Source: CAD feature listing. Evaluate the final solid. Frame: model axes, mm. A direction names the side the tool comes from. Give positions to 0.01 mm unless a question says otherwise; leave off trailing zeros. Loops run counter-clockwise (first coordinate to the right, second up) from the corner with the lowest first, then second, coordinate; pieces in that order, holes last. Notation, with made-up numbers: M 40.25,60 L 47.25,60 A23 ccw 47.25,76 Z; hole C 70,-17 d6. An arc over 180 degrees is marked long. Write item = value, one per line.
Autodesk Inventor part; units mm, degrees
ref_plane "YZ Plane" through (0, 0, 0) normal (1, 0, 0) x (0, 1, 0)
ref_plane "XZ Plane" through (0, 0, 0) normal (0, 1, 0) x (-1, 0, 0)
ref_plane "XY Plane" through (0, 0, 0) normal (0, 0, 1) x (1, 0, 0)
sketch "Sketch1" plane through (0, 0, 0) normal (0, 0, 1) x (1, 0, 0)
  line L0 (-25, 25) -> (25, 25)
  line L1 (25, 25) -> (25, -25)
  line L2 (25, -25) -> (-25, -25)
  line L3 (-25, -25) -> (-25, 25)
  line L4 (-25, 25) -> (25, -25) construction
  line L5 (25, 25) -> (-25, -25) construction
  circle A0 centre (0, 0) radius 2.5
  circle A1 centre (-20.8, -14.5) radius 2.65
  circle A2 centre (-14.5, -20.8) radius 2.65
  circle A3 centre (-20.8, 14.5) radius 2.65
  circle A4 centre (20.8, -14.5) radius 2.65
  circle A5 centre (20.8, 14.5) radius 2.65
  circle A6 centre (-14.5, 20.8) radius 2.65
  circle A7 centre (14.5, -20.8) radius 2.65
  circle A8 centre (14.5, 20.8) radius 2.65
  dimension "d0" = 50
  dimension "d1" = 50
  dimension "d2" = 5
  dimension "d5" = 5.3
  dimension "d6" = 4.2
  dimension "d8" = 10.5
  dimension "d11" = 29
  dimension "d14" = 41.6
extrude "Extrusion1" add sketch "Sketch1" along normal blind 5
fillet "Fillet1" radius 2 4 edges at (-25, 25, 2.5) (25, 25, 2.5) (-25, -25, 2.5) (25, -25, 2.5)
sketch "Sketch2" plane through (0, 0, 5) normal (0, 0, 1) x (1, 0, 0)
  arc A0 (23, -25) -> (25, -23) centre (23, -23) ccw
  line L0 (25, -23) -> (25, 23)
  arc A1 (25, 23) -> (23, 25) centre (23, 23) ccw
  line L1 (23, 25) -> (-23, 25)
  arc A2 (-23, 25) -> (-25, 23) centre (-23, 23) ccw
  line L2 (-25, 23) -> (-25, -23)
  arc A3 (-25, -23) -> (-23, -25) centre (-23, -23) ccw
  line L3 (-23, -25) -> (23, -25)
  circle A4 centre (14.5, 20.8) radius 2.65
  circle A5 centre (-14.5, 20.8) radius 2.65
  circle A6 centre (14.5, -20.8) radius 2.65
  circle A7 centre (20.8, 14.5) radius 2.65
  circle A8 centre (20.8, -14.5) radius 2.65
  circle A9 centre (-20.8, 14.5) radius 2.65
  circle A10 centre (-14.5, -20.8) radius 2.65
  circle A11 centre (-20.8, -14.5) radius 2.65
  circle A12 centre (0, 0) radius 2.5
  line L4 (21, -21) -> (-21, -21)
  line L5 (-21, -21) -> (-21, 21)
  line L6 (-21, 21) -> (21, 21)
  line L7 (21, 21) -> (21, -21)
  line L8 (21, -21) -> (-21, 21) construction
  line L9 (-21, -21) -> (21, 21) construction
  circle A13 centre (-28.6, 21.06) radius 1.55
  dimension "d18" = 42
  dimension "d19" = 42
hole "Hole1" at (-21, 21, 5) at (21, 21, 5) at (21, -21, 5) at (-21, -21, 5) direction (0, 0, -1) diameter 3.3 end through all both
sketch "Sketch3" plane through (0, 0, 0) normal (0, 0, -1) x (-1, 0, 0)
  circle A0 centre (-21, -21) radius 1.65 construction
  circle A1 centre (21, 21) radius 1.65 construction
  circle A2 centre (-21, 21) radius 1.65 construction
  circle A3 centre (21, -21) radius 1.65 construction
  circle A4 centre (-14.5, 20.8) radius 2.65 construction
  circle A5 centre (14.5, 20.8) radius 2.65 construction
  circle A6 centre (-14.5, -20.8) radius 2.65 construction
  circle A7 centre (-20.8, 14.5) radius 2.65 construction
  circle A8 centre (-20.8, -14.5) radius 2.65 construction
  circle A9 centre (20.8, 14.5) radius 2.65 construction
  circle A10 centre (14.5, -20.8) radius 2.65 construction
  circle A11 centre (20.8, -14.5) radius 2.65 construction
  circle A12 centre (0, 0) radius 2.5 construction
  arc A13 (-25, -23) -> (-23, -25) centre (-23, -23) ccw construction
  line L0 (-23, -25) -> (23, -25) construction
  arc A14 (23, -25) -> (25, -23) centre (23, -23) ccw construction
  line L1 (25, -23) -> (25, 23) construction
  arc A15 (25, 23) -> (23, 25) centre (23, 23) ccw construction
  line L2 (23, 25) -> (-23, 25) construction
  arc A16 (-23, 25) -> (-25, 23) centre (-23, 23) ccw construction
  line L3 (-25, 23) -> (-25, -23) construction
  circle A17 centre (-7.5, 7.5) radius 0.9 construction
  circle A18 centre (7.5, 7.5) radius 0.9 construction
  circle A19 centre (7.5, -7.5) radius 0.9 construction
  circle A20 centre (-7.5, -7.5) radius 0.9 construction
hole "Hole2" at (7.5, 7.5, 0) at (-7.5, 7.5, 0) at (-7.5, -7.5, 0) at (7.5, -7.5, 0) direction (0, 0, 1) diameter 1.8 end through all
sketch "Sketch4" plane through (0, 0, 0) normal (0, 0, -1) x (-1, 0, 0)
  line L0 (15, 15) -> (15, -15) construction
  line L1 (-15, 15) -> (15, 15) construction
  line L2 (15, -15) -> (-15, -15) construction
  line L3 (-15, -15) -> (-15, 15) construction
  circle A0 centre (7.5, -7.5) radius 0.9 construction
  circle A1 centre (-7.5, 7.5) radius 0.9 construction
  circle A2 centre (7.5, 7.5) radius 0.9 construction
  circle A3 centre (-7.5, -7.5) radius 0.9 construction
  circle A4 centre (-21, -21) radius 1.65 construction
  circle A5 centre (21, 21) radius 1.65 construction
  circle A6 centre (-21, 21) radius 1.65 construction
  circle A7 centre (21, -21) radius 1.65 construction
  circle A8 centre (-14.5, 20.8) radius 2.65 construction
  circle A9 centre (14.5, 20.8) radius 2.65 construction
  circle A10 centre (-14.5, -20.8) radius 2.65 construction
  circle A11 centre (-20.8, 14.5) radius 2.65 construction
  circle A12 centre (-20.8, -14.5) radius 2.65 construction
  circle A13 centre (20.8, 14.5) radius 2.65 construction
  circle A14 centre (14.5, -20.8) radius 2.65 construction
  circle A15 centre (20.8, -14.5) radius 2.65 construction
  circle A16 centre (0, 0) radius 2.5 construction
  arc A17 (-25, -23) -> (-23, -25) centre (-23, -23) ccw construction
  line L4 (-23, -25) -> (23, -25) construction
  arc A18 (23, -25) -> (25, -23) centre (23, -23) ccw construction
  line L5 (25, -23) -> (25, 23) construction
  arc A19 (25, 23) -> (23, 25) centre (23, 23) ccw construction
  line L6 (23, 25) -> (-23, 25) construction
  arc A20 (-23, 25) -> (-25, 23) centre (-23, 23) ccw construction
  line L7 (-25, 23) -> (-25, -23) construction
  line L8 (-25, -23) -> (-25, 23) construction
  line L9 (-25, 0) -> (25, 0) construction
  line L10 (25, 23) -> (25, -23) construction
  line L11 (10, 6) -> (15, 6) construction
  line L12 (15, 6) -> (15, -6) construction
  line L13 (15, -6) -> (10, -6) construction
  line L14 (10, -6) -> (10, 6) construction
  line L15 (10, 6) -> (25, 6)
  line L16 (25, 6) -> (25, -6)
  line L17 (25, -6) -> (10, -6)
  line L18 (10, -6) -> (10, 6)
  dimension "d34" = 5
  dimension "d35" = 12
extrude "Extrusion2" cut sketch "Sketch4" against normal blind 3
sketch "Sketch5" plane through (0, 0, 3) normal (0, 0, -1) x (-1, 0, 0)
  line L0 (10, 6) -> (25, 6)
  line L1 (10, -6) -> (10, 6)
  line L2 (25, -6) -> (10, -6)
  line L3 (25, 6) -> (25, -6)
  line L4 (25, 6) -> (25, -6)
  line L5 (25, -6) -> (10, -6)
  line L6 (25, 6) -> (22, 6)
  line L7 (22, 6) -> (22, -6)
  line L8 (22, -6) -> (25, -6)
  line L9 (25, -6) -> (25, 6)
  point P0 (0, 0)
  dimension "d38" = 3
extrude "Extrusion3" cut sketch "Sketch5" against normal up to surface (2 mm away) contours L0 L3 L2 L7
fillet "Fillet2" radius 1.5 4 edges at (-25, 6, 2.5) (-25, -6, 2.5) (-22, 6, 4) (-22, -6, 4)
properties part number "20_IM_LED_holder"
1. Cut plane D-D, the plane y = 0. Return the cut outline in (x, z).
Derived:
outline = M -22,3 L -10,3 L -10,0 L -2.5,0 L -2.5,5 L -22,5 Z; M 2.5,0 L 25,0 L 25,5 L 2.5,5 Z
2. Material intervals for probe 1 along Y at (x, z) = (14.5, 1.3); probe 2 along Y at (x, z) = (-20.8, 2.25); probe 3 along Y at (x, z) = (21, 0.65), sorted ascending. Write a range as from..to.
Derived:
probe_1 = -25..-23.45, -18.15..18.15, 23.45..25
probe_2 = -25..-22.64, -19.36..-17.15, -11.85..-6, 6..11.85, 17.15..19.36, 22.64..25
probe_3 = -25..-22.65, -19.35..-17.14, -11.86..11.86, 17.14..19.35, 22.65..25
3. Cut plane A-A, the plane x = 7.5. Return the cut outline in (y, z).
Derived:
outline = M -25,0 L -8.4,0 L -8.4,5 L -25,5 Z; M -6.6,0 L 6.6,0 L 6.6,5 L -6.6,5 Z; M 8.4,0 L 25,0 L 25,5 L 8.4,5 Z
4. Cut plane B-B, the plane y = -14.5. Return the cut outline in (x, z), then the cut area to 3 significant figures.
Derived:
outline = M -25,0 L -23.45,0 L -23.45,5 L -25,5 Z; M -18.15,0 L 18.15,0 L 18.15,5 L -18.15,5 Z; M 23.45,0 L 25,0 L 25,5 L 23.45,5 Z
area = 197 mm²
5. Cut plane C-C, the plane z = 1.35. Count the separate pieces of the cut face and the enclosed holes in it, then the cut area to 3 significant figures.
Derived:
separate_pieces = 1
enclosed_holes = 17
area = 2,080 mm²
6. Pull-direction query (Y, two-part tool) for faces 1 (the flat face through (-22, 0, 4)), 2 (the flat face through (0, 6, 5)), 3 (the cylindrical face through (24.43, 24.4, 2.54)); classes: +Y half, -Y half, draft (parallel to the pull), parting line (faces both ways), or undercut.
Derived:
face_1 = undercut
face_2 = draft
face_3 = +Y half
7. Reachability of faces 4 (the flat face through (-10, 0, 1)), 5 (the cylindrical face through (-22.903, -12.888, 2.465)), 6 (the cylindrical face through (-24.55, 6.43, 2.46)) from +Z, -Z, +X, -X, +Y, -Y: full face, straight path, thin tool, end or side. Return the list, or none.
Derived:
face_4 = -Z, -X
face_5 = +Z, -Z
face_6 = +Z, -Z, -X
